Model file for the job. Use its own axes, mm. Face numbers are marked on the shaded views. A direction names the side the tool comes from. Round coordinates to 2 decimals unless told otherwise and drop trailing zeros. Loops run counter-clockwise (first coordinate to the right, second up) from the corner with the lowest first, then second, coordinate; pieces in that order, holes last. Notation, with made-up numbers: M 68.25,78.5 L 124.25,78.5 A36 cw 124.25,116.5 Z; hole C 52.5,54 d3. An arc over 180 degrees is marked long. Answer in a Markdown table with one row per item.
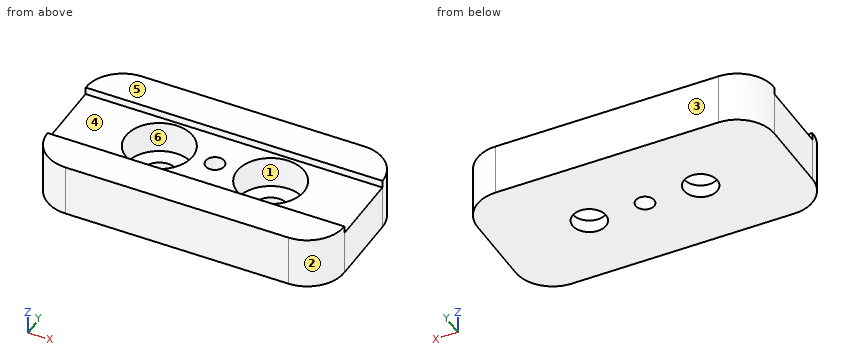
from build123d import *

# Parameters (mm, degrees)
SKETCH_1_W                   = 80
SKETCH_1_H                   = 40
EXTRUDE_1_DEPTH              = 14
SKETCH_2_W                   = 80
SKETCH_2_H                   = 20
CUT_EXTRUDE_1_DEPTH          = 2
HOLE_WIZARD_M6_1_D           = 5
HOLE_WIZARD_M6_1_DEPTH       = 15
HOLE_WIZARD_M6_1_TIP         = 1.502151548
HOLE_WIZARD_M8_1_D           = 9
HOLE_WIZARD_M8_1_CBORE_D     = 18
HOLE_WIZARD_M8_1_CBORE_DEPTH = 8.5
FILLET_1_R                   = 10


with BuildPart() as part:
    # 草图1 → 凸台-拉伸1 (new body)
    with BuildSketch(Plane.XY):
        Rectangle(SKETCH_1_W, SKETCH_1_H)
    extrude(amount=EXTRUDE_1_DEPTH)

    # 草图2 → 切除-拉伸1 (cut)
    with BuildSketch(Plane.XY.offset(14)):
        Rectangle(SKETCH_2_W, SKETCH_2_H)
    extrude(amount=-CUT_EXTRUDE_1_DEPTH, mode=Mode.SUBTRACT)

    # M6 螺纹孔1
    with Locations(Plane.XY.offset(12)):
        with Locations((0, 0)):
            Hole(HOLE_WIZARD_M6_1_D / 2, depth=HOLE_WIZARD_M6_1_DEPTH)
            with Locations((0, 0, -(HOLE_WIZARD_M6_1_DEPTH + HOLE_WIZARD_M6_1_TIP / 2))):  # 118° drill point
                Cone(0, HOLE_WIZARD_M6_1_D / 2, HOLE_WIZARD_M6_1_TIP, mode=Mode.SUBTRACT)

    # M8 六角头螺栓的柱形沉头孔1 (through all)
    with Locations(Plane.XY.offset(12)):
        with Locations((-15, 0), (15, 0)):
            CounterBoreHole(HOLE_WIZARD_M8_1_D / 2, HOLE_WIZARD_M8_1_CBORE_D / 2, HOLE_WIZARD_M8_1_CBORE_DEPTH)

    # 圆角1
    fillet_1_edges = [part.edges().sort_by_distance(p)[0] for p in [
        (-40, 20, 7),
        (40, 20, 7),
        (40, -20, 7),
        (-40, -20, 7),
    ]]
    fillet(fillet_1_edges, radius=FILLET_1_R - 0.0001)  # a hair under: the kernel refuses the full size


solid = part.part
1. Tool access for the marked faces 1 and 2: list every direction of +Z, -Z, +X, -X, +Y, -Y with a clear straight run to the whole face (end or side of a thin tool).
Verdict:
| item | result |
|---|---|
| face 1 | +Z |
| face 2 | +Z, -Z, +X, -Y |
2. Saw through at C-C (x = 15). Write the cut outline in (y, z).
Verdict:
| item | result |
|---|---|
| outline | M -20,0 L -4.5,0 L -4.5,3.5 L -9,3.5 L -9,12 L -10,12 L -10,14 L -20,14 Z; M 4.5,0 L 20,0 L 20,14 L 10,14 L 10,12 L 9,12 L 9,3.5 L 4.5,3.5 Z |
3. Pin check, flat tips, straight feed: pin 1 (1 mm diameter, centred on x = 17, y = -6.5, fed in from +Z); pin 2 (3 mm diameter, centred on y = 13.5, z = 5.5, fed in from -X); pin 3 (22 mm diameter, centred on x = 7.5, y = 5, fed in from +Z); pin 4 (6 mm diameter, centred on x = 0, y = 0, fed in from +Z). Stop position of each tip, or through.
Verdict:
| item | result |
|---|---|
| pin 1 | stops at z = 3.5 |
| pin 2 | stops at x = -39.8 |
| pin 3 | stops at z = 14 |
| pin 4 | stops at z = 12 |
4. Mould opens along Y. For the marked faces 3, 4, 5 and 6 say: +Y half, -Y half, draft (parallel to the pull), parting line (faces both ways), or undercut.
Verdict:
| item | result |
|---|---|
| face 3 | +Y half |
| face 4 | undercut |
| face 5 | draft |
| face 6 | undercut |
5. Wall check: probe 1 along Y at (x, z) = (15, 2.5); probe 2 along X at (y, z) = (-7, 11.75); probe 3 along Y at (x, z) = (15, 5.75). Give the ranges that are in metal, low to high.
Verdict:
| item | result |
|---|---|
| probe 1 | y = -20 to -4.5, 4.5 to 20 |
| probe 2 | x = -40 to -20.66, -9.34 to 9.34, 20.66 to 40 |
| probe 3 | y = -20 to -9, 9 to 20 |
6. Saw through at D-D (y = 6). Write the cut outline in (x, z).
Verdict:
| item | result |
|---|---|
| outline | M -40,0 L 40,0 L 40,12 L 21.71,12 L 21.71,3.5 L 8.29,3.5 L 8.29,12 L -8.29,12 L -8.29,3.5 L -21.71,3.5 L -21.71,12 L -40,12 Z |
7. Saw through at A-A (x = 0). Write the cut outline in (y, z), and give its area (3 significant figures).
Verdict:
| item | result |
|---|---|
| outline | M -20,0 L -2.5,0 L -2.5,12 L -10,12 L -10,14 L -20,14 Z; M 2.5,0 L 20,0 L 20,14 L 10,14 L 10,12 L 2.5,12 Z |
| area | 460 mm² |
8. Saw through at B-B (y = 1.5). Write the cut outline in (x, z).
Verdict:
| item | result |
|---|---|
| outline | M -40,0 L -19.24,0 L -19.24,3.5 L -23.87,3.5 L -23.87,12 L -40,12 Z; M -10.76,0 L -2,0 L -2,12 L -6.13,12 L -6.13,3.5 L -10.76,3.5 Z; M 2,0 L 10.76,0 L 10.76,3.5 L 6.13,3.5 L 6.13,12 L 2,12 Z; M 19.24,0 L 40,0 L 40,12 L 23.87,12 L 23.87,3.5 L 19.24,3.5 Z |
